Study the drawing (mm; zero at the part's minimum x, y, z) and answer. A direction names the side the tool comes from. Give positions to 0.01 mm unless a question says otherwise; leave off trailing zeros. Order: outer loops, then holes, each group sorted by start corner. A loop starts at its lowest first (then second) coordinate and runs counter-clockwise, first axis right, second up. Notation, with made-up numbers: (2.25, -25) - (25.25, -25) arc R20 cw to (25.25, 3) - close; hole circle Ø6 at (31.25, -8.75). An arc over 180 degrees is marked (long way). Return JSON: item names as keys, results as strings.
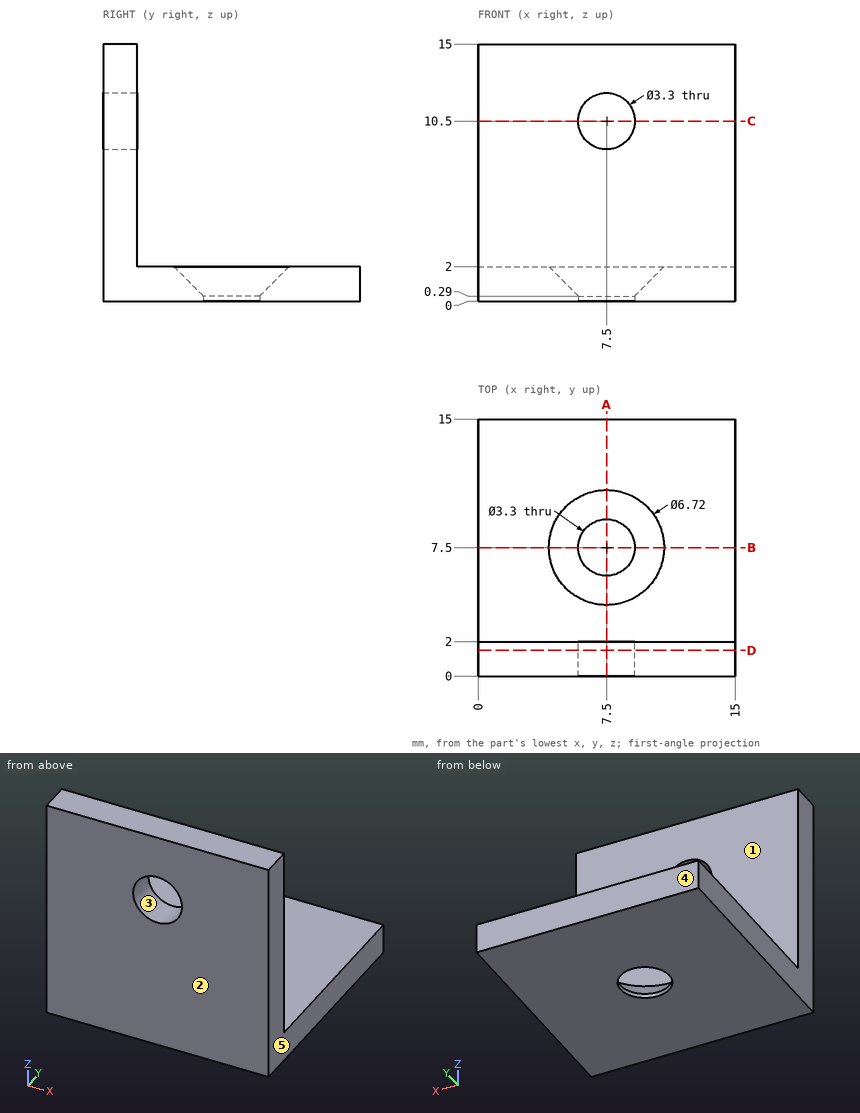
Q1. A cutting plane is placed at C-C (z = 10.5). Write down the section's boundary in (x, y).
Values:
{"outline": "(0, 0) - (5.85, 0) - (5.85, 2) - (0, 2) - close; (9.15, 0) - (15, 0) - (15, 2) - (9.15, 2) - close"}
Q2. Determine the mould class of the marked faces 3, 4 and 5 for opening direction X: released by +X, released by -X, zero draft, split by the parting line, or undercut.
Values:
{"face 3": "undercut", "face 4": "zero draft", "face 5": "released by +X"}
Q3. A cutting plane is placed at A-A (x = 7.5). Write down the section's boundary in (y, z), and give its area (3 significant figures).
Values:
{"outline": "(0, 0) - (5.85, 0) - (5.85, 0.29) - (4.14, 2) - (2, 2) - (2, 8.85) - (0, 8.85) - close; (0, 12.15) - (2, 12.15) - (2, 15) - (0, 15) - close; (9.15, 0) - (15, 0) - (15, 2) - (10.86, 2) - (9.15, 0.29) - close", "area": "39.9 mm²"}
Q4. Consider L1, parallel to X at y = 7.5, z = 0.25; L2, parallel to Y at x = 1.5, z = 4.75. Determine where each line is inside the solid, lowest interval first.
Values:
{"L1": "x = 0 to 5.85, 9.15 to 15", "L2": "y = 0 to 2"}
Q5. A cutting plane is placed at D-D (y = 1.5). Write down the section's boundary in (x, z), and give its area (3 significant figures).
Values:
{"outline": "(0, 0) - (15, 0) - (15, 15) - (0, 15) - close; hole circle Ø3.3 at (7.5, 10.5)", "area": "216 mm²"}
Q6. Given pin 1 (4 mm diameter, centred on x = 9, y = 10.5, fed in from +Z); pin 2 (1 mm diameter, centred on x = 8, y = 7.5, fed in from +Z); pin 3 (4 mm diameter, centred on x = 9, z = 11.5, fed in from +Y), each flat-ended and moving along its own axis, determine where each tip first touches the part or whether it passes through.
Values:
{"pin 1": "stops at z = 2", "pin 2": "passes through", "pin 3": "stops at y = 2"}
Q7. A cutting plane is placed at B-B (y = 7.5). Write down the section's boundary in (x, z), and give its area (3 significant figures).
Values:
{"outline": "(0, 0) - (5.85, 0) - (5.85, 0.29) - (4.14, 2) - (0, 2) - close; (9.15, 0) - (15, 0) - (15, 2) - (10.86, 2) - (9.15, 0.29) - close", "area": "20.5 mm²"}
Q8. For the marked faces 1 and 2, determine the directions among +Z, -Z, +X, -X, +Y, -Y from which every point of the face is accessible in a straight line to the end or side of a thin tool.
Values:
{"face 1": "+Z, +X, -X, +Y", "face 2": "+Z, -Z, +X, -X, -Y"}
